from build123d import *

# Parameters (mm, degrees)
BOX025_W        = 11.5
BOX025_H        = 11.5
BOX025_DEPTH    = 2
BOX023_W        = 11.5
BOX023_H        = 4.45
BOX023_DEPTH    = 7
BOX022_W        = 11.5
BOX022_H        = 4.45
BOX022_DEPTH    = 7
CHAMFER003_SIZE = 1
FILLET008_R     = 1.99


with BuildPart() as beltclipbase:
    # Box025 → Box025 (new body)
    with BuildSketch(Plane(origin=(40, 9, 14), x_dir=(1, 0, 0), z_dir=(0, 0, 1))):
        with Locations((5.75, 5.75)):
            Rectangle(BOX025_W, BOX025_H)
    extrude(amount=BOX025_DEPTH)


with BuildPart() as beltclipright:
    # Box023 → Box023 (new body)
    with BuildSketch(Plane(origin=(40, 16.05, 16), x_dir=(1, 0, 0), z_dir=(0, 0, 1))):
        with Locations((5.75, 2.225)):
            Rectangle(BOX023_W, BOX023_H)
    extrude(amount=BOX023_DEPTH)


with BuildPart() as belt_clip:
    # Box022 → Box022 (new body)
    with BuildSketch(Plane(origin=(40, 9, 16), x_dir=(1, 0, 0), z_dir=(0, 0, 1))):
        with Locations((5.75, 2.225)):
            Rectangle(BOX022_W, BOX022_H)
    extrude(amount=BOX022_DEPTH)

    # Fusion030: union BeltClipBase, BeltClipRight
    add(beltclipbase.part)
    add(beltclipright.part)

    # Chamfer003
    chamfer003_edges = [belt_clip.edges().sort_by_distance(p)[0] for p in [
        (45.75, 16.05, 23),
        (45.75, 13.45, 23),
    ]]
    chamfer(chamfer003_edges, length=CHAMFER003_SIZE)

    # Fillet008
    fillet008_edges = [belt_clip.edges().sort_by_distance(p)[0] for p in [
        (40, 20.5, 19.5),
        (51.5, 20.5, 19.5),
        (40, 14.75, 14),
        (45.75, 20.5, 14),
        (51.5, 14.75, 14),
        (45.75, 9, 14),
        (40, 9, 19.5),
        (51.5, 9, 19.5),
    ]]
    fillet(fillet008_edges, radius=FILLET008_R)


with BuildPart() as belt_clip_1:
    # Fillet008 placement: moved
    add(belt_clip.part.moved(Location((18, 2, 0))))


solid = belt_clip_1.part
Source: CAD feature listing. Evaluate the final solid. Frame: model axes, mm. A direction names the side the tool comes from. Give positions to 0.01 mm unless a question says otherwise; leave off trailing zeros. Write each loop counter-clockwise with the first axis right and the second up, starting at its lowest first coordinate (ties: lowest second). Pieces come first, ordered by that corner, then holes. Notation, with made-up numbers: (5.5, 73) -> (26.5, 73) arc R15 cw to (26.5, 94) -> close; hole circle Ø1 at (86.5, -19). An arc over 180 degrees is marked (long way). Write item = value, one per line.
Q1. First-contact query: pin 1 (4 mm diameter, centred on y = 18, z = 15, fed in from -X); pin 2 (1.3 mm diameter, centred on x = 61.5, y = 16.5, fed in from +Z). Flat tips, straight axial feed; report the tip coordinate or a pass-through.
Here are the results:
pin_1 = 58
pin_2 = 16
Q2. Mould query, pull axis Y, two halves, no side actions, for faces 1 (the face through (68.902, 11.567, 19.544)), 2 (the face through (69.5, 15, 19)), 3 (the face through (63.67, 18.54, 22.49)). Classes: +Y half, -Y half, draft (parallel to the pull), parting line (faces both ways), or undercut.
Here are the results:
face_1 = -Y half
face_2 = draft
face_3 = undercut
Q3. Cut plane A-A on z = 17. Return loops of the section in (x, y), then the cut area to 3 significant figures.
Here are the results:
outline = (58, 12.99) arc R1.99 ccw to (59.99, 11) -> (67.51, 11) arc R1.99 ccw to (69.5, 12.99) -> (69.5, 15.45) -> (58, 15.45) -> close; (58, 18.05) -> (69.5, 18.05) -> (69.5, 20.51) arc R1.99 ccw to (67.51, 22.5) -> (59.99, 22.5) arc R1.99 ccw to (58, 20.51) -> close
area = 99.0 mm²
Q4. Cut plane B-B on x = 63.25. Return loops of the section in (y, z), then the cut area to 3 significant figures.
Here are the results:
outline = (11, 15.99) arc R1.99 ccw to (12.99, 14) -> (20.51, 14) arc R1.99 ccw to (22.5, 15.99) -> (22.5, 23) -> (19.05, 23) -> (18.05, 22) -> (18.05, 16) -> (15.45, 16) -> (15.45, 22) -> (14.45, 23) -> (11, 23) -> close
area = 82.6 mm²
Q5. Cut plane D-D on z = 22.25. Return loops of the section in (x, y).
Here are the results:
outline = (58, 12.99) arc R1.99 ccw to (59.99, 11) -> (67.51, 11) arc R1.99 ccw to (69.5, 12.99) -> (69.5, 15.2) -> (58, 15.2) -> close; (58, 18.3) -> (69.5, 18.3) -> (69.5, 20.51) arc R1.99 ccw to (67.51, 22.5) -> (59.99, 22.5) arc R1.99 ccw to (58, 20.51) -> close
Q6. Line query: line 1 (Y direction, x = 61.25, z = 19.5); line 2 (Y direction, x = 58.75, z = 21.25); line 3 (Z direction, x = 61, y = 17). Output: solid intervals per line, ascending. Write a range as from..to.
Here are the results:
line_1 = 11..15.45, 18.05..22.5
line_2 = 11.43..15.45, 18.05..22.07
line_3 = 14..16
Q7. Cut plane C-C on y = 13.75. Return loops of the section in (x, z).
Here are the results:
outline = (58, 15.99) arc R1.99 ccw to (59.99, 14) -> (67.51, 14) arc R1.99 ccw to (69.5, 15.99) -> (69.5, 23) -> (58, 23) -> close
Q8. Reachability of faces 4 (the face through (63.803, 21.933, 14.598)), 5 (the face through (64, 17, 16)) from +Z, -Z, +X, -X, +Y, -Y: full face, straight path, thin tool, end or side. Return the list, or none.
Here are the results:
face_4 = -Z, +X, -X, +Y
face_5 = +Z, +X, -X
